Geometry: see drawing. Coordinates: mm, zero at the bounding-box minimum. Give positions to 0.01 mm unless a question says otherwise; leave off trailing zeros. Order: outer loops, then holes, each group sorted by start corner. A loop starts at its lowest first (then second) coordinate and runs counter-clockwise, first axis right, second up. Notation, with made-up numbers: (46, 30.5) -> (64, 30.5) arc R36 ccw to (64, 64.5) -> close; hole circle Ø2 at (-7, 50.5). An arc over 180 degrees is marked (long way). One line per item, written item: value. Start each with the question number.
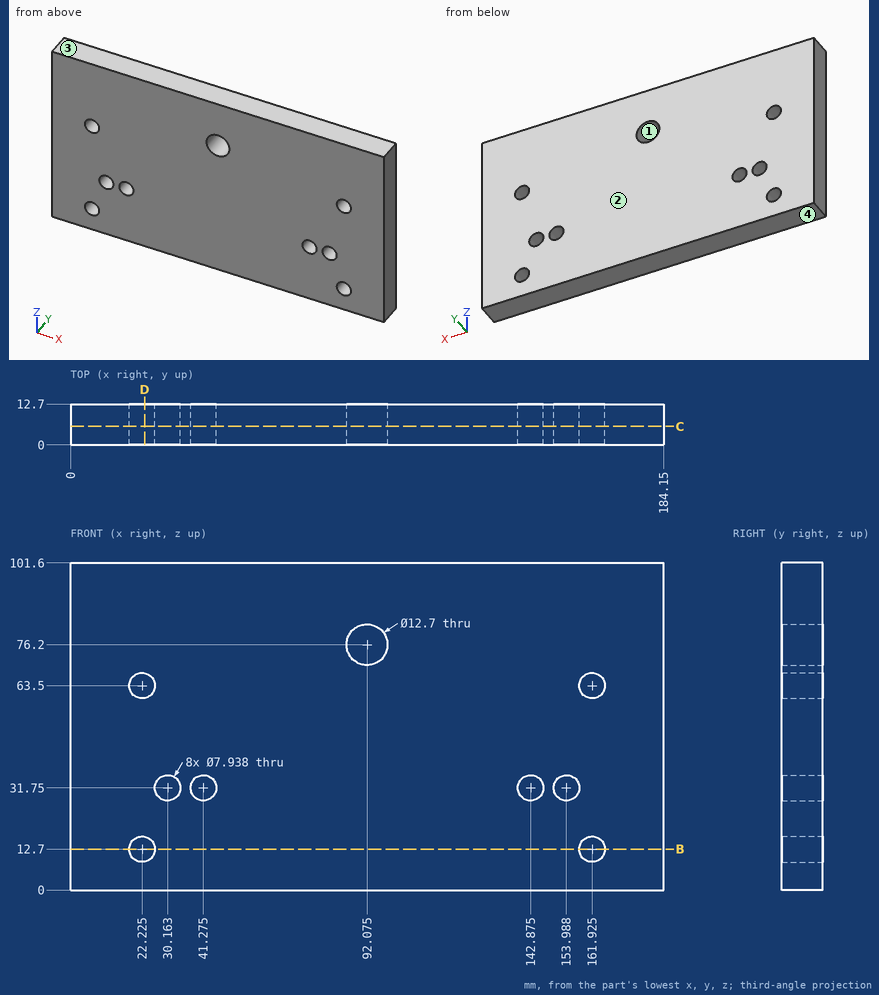
1. Draft query along Z for the marked faces 1, 2, 3 and 4. Return one class per face: pulls with the +Z half, pulls with the -Z half, needs draft (parallel to the pull), parting line crosses it, or undercut.
2. Cut plane C-C, the plane y = 5.75. State how many separate pieces and enclosed holes the cut face has, then the cut area to 3 significant figures.
3. Material intervals for L1, parallel to X at y = 8.25, z = 12.5; L2, parallel to Z at x = 160.5, y = 4.5 (1 decimal); L3, parallel to Z at x = 30, y = 7.5 (1 decimal), sorted ascending. Write a range as [from, to].
4. Pin query (flat end, axial travel): P1, Ø12.5, axis at x = 153.99, z = 31.75, coming from the -Y side; P2, Ø6.5, axis at x = 142.875, z = 31.75, coming from the -Y side. Return the tip coordinate at first contact, or that it passes through.
5. Cut plane B-B, the plane z = 12.7. Return loops of the section in (x, y).
6. Cut plane D-D, the plane x = 23. Return loops of the section in (y, z), then the cut area to 3 significant figures.
Answers follow:
1. face 1: undercut
1. face 2: needs draft
1. face 3: pulls with the +Z half
1. face 4: pulls with the -Z half
2. separate pieces: 1
2. enclosed holes: 9
2. area: 18,200 mm²
3. L1: x = [0, 18.26], [26.19, 157.96], [165.89, 184.15]
3. L2: z = [0, 9], [16.4, 59.8], [67.2, 101.6]
3. L3: z = [0, 27.8], [35.7, 101.6]
4. P1: stops at y = 0
4. P2: passes through
5. outline: (0, 0) -> (18.26, 0) -> (18.26, 12.7) -> (0, 12.7) -> close; (26.19, 0) -> (157.96, 0) -> (157.96, 12.7) -> (26.19, 12.7) -> close; (165.89, 0) -> (184.15, 0) -> (184.15, 12.7) -> (165.89, 12.7) -> close
6. outline: (0, 0) -> (12.7, 0) -> (12.7, 8.81) -> (0, 8.81) -> close; (0, 16.59) -> (12.7, 16.59) -> (12.7, 59.61) -> (0, 59.61) -> close; (0, 67.39) -> (12.7, 67.39) -> (12.7, 101.6) -> (0, 101.6) -> close
6. area: 1,090 mm²
